Geometry check sheet. Reference: drawing and pictorial views, mm from the part's lowest x, y, z. A direction names the side the tool comes from. Give positions to 0.01 mm unless a question says otherwise; leave off trailing zeros. Loops run counter-clockwise (first coordinate to the right, second up) from the corner with the lowest first, then second, coordinate; pieces in that order, holes last. Notation, with made-up numbers: (64.25, -31.5) -> (95.25, -31.5) arc R16 ccw to (95.25, -22.5) -> close; hole circle Ø5 at (21, 82). An arc over 180 degrees is marked (long way). Answer in a Markdown table with one row per item. Add a question column.
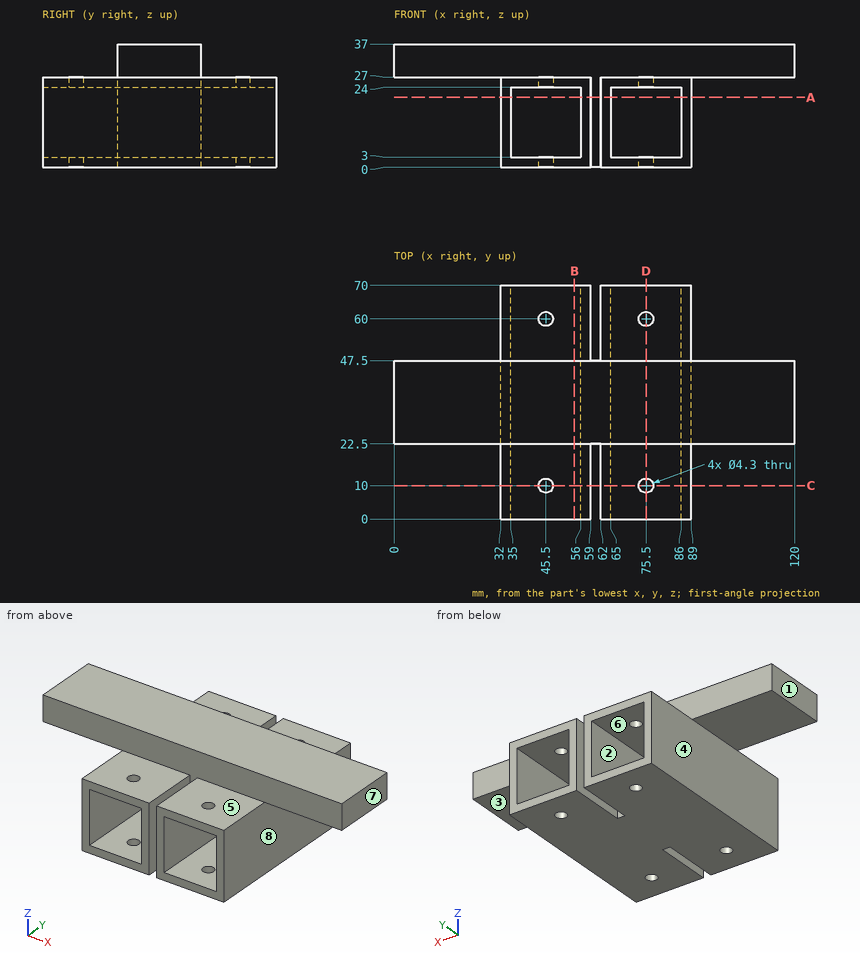
1. Gauge pin test, flat ends, axial feed: pin 1 Ø12.5 at (x, y) = (18.5, 35) entering from -Z; pin 2 Ø4 at (x, y) = (75.5, 60) entering from -Z; pin 3 Ø10.5 at (y, z) = (49, 11.5) entering from +X; pin 4 Ø5.5 at (x, y) = (45.5, 60) entering from +Z. Record the tip position at first contact, or that the pin passes through.
2. Sectioned sample at D-D (x = 75.5). Enter the section's corners in (y, z).
3. Sectioned sample at A-A (z = 21). Enter the section's corners in (x, y), plus the area to 3 significant figures.
4. Sectioned sample at C-C (y = 10). Count the separate pieces of the cut face and the enclosed holes in it, plus the area to 3 significant figures.
5. Access from +Z, -Z, +X, -X, +Y, -Y to the whole of each face (thin tool, end or side, straight path). Record for the marked faces 4, 5, 6, 7 and 8.
6. Material ranges on L1, parallel to X at y = 60.5, z = 7.5; L2, parallel to X at y = 33.5, z = 22.5; L3, parallel to Z at x = 43, y = 12, recorded low to high. Write a range as from..to.
7. Release check for a two-part mould opening along Z. For the marked faces 1, 2 and 3 record: released by +Z, released by -Z, zero draft, split by the parting line, or undercut.
8. Sectioned sample at B-B (x = 54). Enter the section's corners in (y, z), plus the area to 3 significant figures.
Response:
| question | item | result |
|---|---|---|
| 1 | pin 1 | stops at z = 27 |
| 1 | pin 2 | passes through |
| 1 | pin 3 | stops at x = 89 |
| 1 | pin 4 | stops at z = 27 |
| 2 | outline | (0, 0) -> (7.85, 0) -> (7.85, 3) -> (0, 3) -> close; (0, 24) -> (7.85, 24) -> (7.85, 27) -> (0, 27) -> close; (12.15, 0) -> (57.85, 0) -> (57.85, 3) -> (12.15, 3) -> close; (12.15, 24) -> (57.85, 24) -> (57.85, 27) -> (47.5, 27) -> (47.5, 37) -> (22.5, 37) -> (22.5, 27) -> (12.15, 27) -> close; (62.15, 0) -> (70, 0) -> (70, 3) -> (62.15, 3) -> close; (62.15, 24) -> (70, 24) -> (70, 27) -> (62.15, 27) -> close |
| 3 | outline | (32, 0) -> (35, 0) -> (35, 70) -> (32, 70) -> close; (56, 0) -> (59, 0) -> (59, 22.5) -> (62, 22.5) -> (62, 0) -> (65, 0) -> (65, 70) -> (62, 70) -> (62, 47.5) -> (59, 47.5) -> (59, 70) -> (56, 70) -> close; (86, 0) -> (89, 0) -> (89, 70) -> (86, 70) -> close |
| 3 | area | 915 mm2 |
| 4 | separate pieces | 4 |
| 4 | enclosed holes | 0 |
| 4 | area | 524 mm2 |
| 5 | face 4 | -Z, -X, +Y, -Y |
| 5 | face 5 | +Z, +X, -X, -Y |
| 5 | face 6 | +Y, -Y |
| 5 | face 7 | +Z, -Z, +X, +Y, -Y |
| 5 | face 8 | -Z, +X, +Y, -Y |
| 6 | L1 | x = 32..35, 56..59, 62..65, 86..89 |
| 6 | L2 | x = 32..35, 56..65, 86..89 |
| 6 | L3 | z = 0..3, 24..27 |
| 7 | face 1 | zero draft |
| 7 | face 2 | undercut |
| 7 | face 3 | released by -Z |
| 8 | outline | (0, 0) -> (70, 0) -> (70, 3) -> (0, 3) -> close; (0, 24) -> (70, 24) -> (70, 27) -> (47.5, 27) -> (47.5, 37) -> (22.5, 37) -> (22.5, 27) -> (0, 27) -> close |
| 8 | area | 670 mm2 |
